```python
from build123d import *

# Parameters (mm, degrees)
EXTRUDE_1_DEPTH          = 355
SKETCH_2_R               = 1.3
CUT_EXTRUDE_1_DEPTH      = 1
CUT_EXTRUDE_1_DEPTH_BACK = 10.7
SKETCH_2_3_R             = 2.8
SKETCH_2_3_R_2           = 1.3
CUT_EXTRUDE_2_DEPTH      = 1
CUT_EXTRUDE_2_DEPTH_BACK = 4
SKETCH_13_R              = 2.8
SKETCH_13_R_2            = 1.6
CUT_EXTRUDE_11_DEPTH     = 17
SKETCH_13_4_R            = 1.6
CUT_EXTRUDE_12_DEPTH     = 20.2


with BuildPart() as part:
    # 草图1 → 凸台-拉伸1 (new body)
    with BuildSketch(Plane.XY):
        Polygon((-3, 0), (-3, 5.6), (-3, 7.6), (2.6, 7.6), (6.7, 7.6), (6.7, 3.7), (4.7, 3.7), (4.7, 5.7), (-1, 5.7), (-1, 0), (-1, -5.7), (4.7, -5.7), (4.7, -3.7), (6.7, -3.7), (6.7, -7.6), (6.7, -11.6), (-3, -11.6), (-3, -7.6), (-3, -5.6), align=None)
    extrude(amount=EXTRUDE_1_DEPTH)

    # 草图2 → 切除-拉伸1 (cut, two sides)
    with BuildSketch(Plane.ZY.offset(3)) as cut_extrude_1_sk:
        with Locations((150, -8.6)):
            Circle(SKETCH_2_R)
        with Locations((100, -8.6)):
            Circle(SKETCH_2_R)
        with Locations((50, -8.6)):
            Circle(SKETCH_2_R)
        with Locations((200, -8.6)):
            Circle(SKETCH_2_R)
        with Locations((250, -8.6)):
            Circle(SKETCH_2_R)
        with Locations((300, -8.6)):
            Circle(SKETCH_2_R)
        with Locations((350, -8.6)):
            Circle(SKETCH_2_R)
    extrude(amount=CUT_EXTRUDE_1_DEPTH, mode=Mode.SUBTRACT)
    extrude(cut_extrude_1_sk.sketch, amount=-CUT_EXTRUDE_1_DEPTH_BACK, mode=Mode.SUBTRACT)

    # 草图2<3> → 切除-拉伸2 (cut, two sides)
    with BuildSketch(Plane.ZY.offset(3)) as cut_extrude_2_sk:
        with Locations((200, -8.6)):
            Circle(SKETCH_2_3_R)
        with Locations((200, -8.6)):
            Circle(SKETCH_2_3_R_2, mode=Mode.SUBTRACT)
        with Locations((250, -8.6)):
            Circle(SKETCH_2_3_R)
        with Locations((250, -8.6)):
            Circle(SKETCH_2_3_R_2, mode=Mode.SUBTRACT)
        with Locations((150, -8.6)):
            Circle(SKETCH_2_3_R)
        with Locations((150, -8.6)):
            Circle(SKETCH_2_3_R_2, mode=Mode.SUBTRACT)
        with Locations((100, -8.6)):
            Circle(SKETCH_2_3_R)
        with Locations((100, -8.6)):
            Circle(SKETCH_2_3_R_2, mode=Mode.SUBTRACT)
        with Locations((50, -8.6)):
            Circle(SKETCH_2_3_R)
        with Locations((50, -8.6)):
            Circle(SKETCH_2_3_R_2, mode=Mode.SUBTRACT)
        with Locations((300, -8.6)):
            Circle(SKETCH_2_3_R)
        with Locations((300, -8.6)):
            Circle(SKETCH_2_3_R_2, mode=Mode.SUBTRACT)
        with Locations((350, -8.6)):
            Circle(SKETCH_2_3_R)
        with Locations((350, -8.6)):
            Circle(SKETCH_2_3_R_2, mode=Mode.SUBTRACT)
    extrude(amount=CUT_EXTRUDE_2_DEPTH, mode=Mode.SUBTRACT)
    extrude(cut_extrude_2_sk.sketch, amount=-CUT_EXTRUDE_2_DEPTH_BACK, mode=Mode.SUBTRACT)

    # 草图13 → 切除-拉伸11 (cut)
    with BuildSketch(Plane(origin=(0, 7.6, 0), x_dir=(1, 0, 0), z_dir=(0, 1, 0))):
        with Locations((1.8, -10)):
            Circle(SKETCH_13_R)
        with Locations((1.8, -10)):
            Circle(SKETCH_13_R_2, mode=Mode.SUBTRACT)
        with Locations((1.8, -120)):
            Circle(SKETCH_13_R)
        with Locations((1.8, -120)):
            Circle(SKETCH_13_R_2, mode=Mode.SUBTRACT)
        with Locations((1.8, -230)):
            Circle(SKETCH_13_R)
        with Locations((1.8, -230)):
            Circle(SKETCH_13_R_2, mode=Mode.SUBTRACT)
        with Locations((1.8, -340)):
            Circle(SKETCH_13_R)
        with Locations((1.8, -340)):
            Circle(SKETCH_13_R_2, mode=Mode.SUBTRACT)
    extrude(amount=-CUT_EXTRUDE_11_DEPTH, mode=Mode.SUBTRACT)

    # 草图13<4> → 切除-拉伸12 (cut, through all)
    with BuildSketch(Plane(origin=(0, 7.6, 0), x_dir=(1, 0, 0), z_dir=(0, 1, 0))):
        with Locations((1.8, -340)):
            Circle(SKETCH_13_4_R)
        with Locations((1.8, -230)):
            Circle(SKETCH_13_4_R)
        with Locations((1.8, -120)):
            Circle(SKETCH_13_4_R)
        with Locations((1.8, -10)):
            Circle(SKETCH_13_4_R)
    extrude(amount=-CUT_EXTRUDE_12_DEPTH, mode=Mode.SUBTRACT)


solid = part.part
```
Design review of the part built by this model. Coordinates are the model's own, in mm. A direction names the side the tool comes from. Give positions to 0.01 mm unless a question says otherwise; leave off trailing zeros. Order: outer loops, then holes, each group sorted by start corner. A loop starts at its lowest first (then second) coordinate and runs counter-clockwise, first axis right, second up. Notation, with made-up numbers: (80, 64) -> (119, 64) arc R21 ccw to (119, 94) -> close; hole circle Ø6 at (19.5, 83.5). An arc over 180 degrees is marked (long way). Write item = value, one per line. Start each with the question number.
(1) For faces 4 (the face through (2, -9.4, 232)), 5 (the face through (2, 7.6, 175)), 6 (the face through (1, -10, 151)), list the 3-axis set-ups (+Z, -Z, +X, -X, +Y, -Y) from which the entire face can be reached by the end or side of a thin tool; tool diameter is ignored.
(2) For pin 1 (1.5 mm diameter, centred on x = 5.5, y = -8.5, fed in from -Z); pin 2 (1.7 mm diameter, centred on y = -8.5, z = 349, fed in from -X); pin 3 (4.5 mm diameter, centred on x = 1.8, z = 230, fed in from +Y); pin 4 (1.5 mm diameter, centred on y = -1, z = 156.5, fed in from +X), all flat-tipped, find the tip position at first contact; note any pin that passes through.
(3) We need section A-A on z = 84. Write out the cut boundary in (x, y).
(4) To check wall thickness, follow line 1 along X through (y, z) = (6.7, 10); line 2 along X through (y, z) = (-4.75, 53); line 3 along Y through (x, z) = (6.25, 98). State the ranges of each line that lie inside material, in increasing order.
(5) Mouldability with a two-part tool opening along X and no side actions: class faces 1 (the face through (2, -11.6, 175)), 2 (the face through (-3, -2, 175)), 3 (the face through (1.435, -7.524, 337.224)) as +X half, -X half, draft (parallel to the pull), parting line (faces both ways), or undercut.
(6) We need section B-B on y = 0.5. Write out the cut boundary in (x, z).
Numbers:
q1.face_4 = +Y
q1.face_5 = +Z, -Z, +X, -X, +Y
q1.face_6 = -X
q2.pin_1 = 0
q2.pin_2 = 1
q2.pin_3 = -9.4
q2.pin_4 = -1
q3.outline = (-3, -11.6) -> (6.7, -11.6) -> (6.7, -3.7) -> (4.7, -3.7) -> (4.7, -5.7) -> (-1, -5.7) -> (-1, 5.7) -> (4.7, 5.7) -> (4.7, 3.7) -> (6.7, 3.7) -> (6.7, 7.6) -> (-3, 7.6) -> close
q4.line_1 = -3 to -1, 4.6 to 6.7
q4.line_2 = -3 to -1, 4.7 to 6.7
q4.line_3 = -11.6 to -3.7, 3.7 to 7.6
q5.face_1 = draft
q5.face_2 = -X half
q5.face_3 = undercut
q6.outline = (-3, 0) -> (-1, 0) -> (-1, 355) -> (-3, 355) -> close
